Geometry: final body of the model. Coordinates: model frame, mm. Face numbers are marked on the shaded views. A direction names the side the tool comes from. Round coordinates to 2 decimals unless told otherwise and drop trailing zeros. Loops run counter-clockwise (first coordinate to the right, second up) from the corner with the lowest first, then second, coordinate; pieces in that order, holes last. Notation, with made-up numbers: (-31.75, -34) -> (-20.75, -34) arc R24 cw to (-20.75, 5) -> close; hole circle Ø3 at (43.5, 31). An arc over 180 degrees is marked (long way). Answer in a Markdown table with one row per item.
```python
from build123d import *

# Parameters (mm, degrees)
F1_DEPTH = 762
F3_DEPTH = 762.001
F4_DEPTH = 533.4
F6_DEPTH = 469.901
F8_DEPTH = 762
F7_R     = 190.5
F9_DEPTH = 762.0010001


with BuildPart() as f1:
    # F0 (on Front) → F1 (new body)
    with BuildSketch(Plane.XZ):
        with BuildLine():
            ThreePointArc((0, 6.35), (1.8598719395, 1.8598719395), (6.35, 0))
            Line((6.35, 0), (1524, 0))
            Line((1524, 0), (1524, 762))
            Line((1524, 762), (6.35, 762))
            ThreePointArc((6.35, 762), (1.8598719395, 760.1401280605), (0, 755.65))
            Line((0, 755.65), (0, 6.35))
        make_face()
    extrude(amount=F1_DEPTH)

    # F2 (on face) → F3 (cut, through all)
    with BuildSketch(Plane.XY.offset(762)):
        Polygon((1524, -228.6), (1524, 0), (1295.4, 0), align=None)
        Polygon((1524, -762), (1524, -533.4), (1295.4, -762), align=None)
    extrude(amount=-F3_DEPTH, mode=Mode.SUBTRACT)

    # F2 (on face) → F4 (cut)
    with BuildSketch(Plane.XY.offset(762)):
        Polygon((1524, -292.1), (1524, -228.6), (1295.4, 0), (457.2, 0), (457.2, -292.1), align=None)
        Polygon((1524, -533.4), (1524, -469.9), (457.2, -469.9), (457.2, -762), (1295.4, -762), align=None)
    extrude(amount=-F4_DEPTH, mode=Mode.SUBTRACT)

    # F5 (on face) → F6 (cut, through all)
    with BuildSketch(Plane.XZ.offset(469.9)):
        Polygon((1524, 762), (457.2, 762), (1524, 228.6), align=None)
    extrude(amount=-F6_DEPTH, mode=Mode.SUBTRACT)

    # F7 (on face) → F8 (join)
    with BuildSketch(Plane.XY.offset(762)):
        with BuildLine():
            Line((6.35, -190.5), (6.35, 0))
            ThreePointArc((6.35, 0), (-374.65, -381), (6.35, -762))
            Line((6.35, -762), (6.35, -571.5))
            ThreePointArc((6.35, -571.5), (-184.15, -381), (6.35, -190.5))
        make_face()
    extrude(amount=-F8_DEPTH)

    # F7 (on face) → F9 (cut, through all)
    with BuildSketch(Plane.XY.offset(762)):
        with Locations((6.35, -381)):
            Circle(F7_R)
    extrude(amount=-F9_DEPTH, mode=Mode.SUBTRACT)


solid = f1.part
```
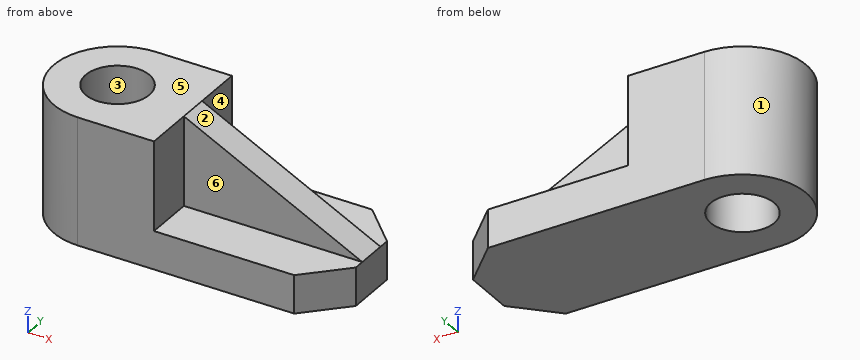
Item 1: First-contact query: P1, Ø2, axis at x = 792.5, z = 431.5, coming from the -Y side; P2, Ø3, axis at x = 1235, y = -614, coming from the +Z side; P3, Ø1, axis at y = -278, z = 478, coming from the +X side. Flat tips, straight axial feed; report the tip coordinate or a pass-through.
Ans:
| item | result |
|---|---|
| P1 | y = -469.9 |
| P2 | z = 228.6 |
| P3 | x = 457.2 |
Item 2: Section query D-D, the plane z = 546. Output: boundary loops of the cut face in (x, y).
Ans:
| item | result |
|---|---|
| outline | (0, -762) -> (457.2, -762) -> (457.2, -469.9) -> (889.2, -469.9) -> (889.2, -292.1) -> (457.2, -292.1) -> (457.2, 0) -> (0, 0) -> (0, -0.05) arc R381 ccw to (0, -761.95) -> close; hole circle Ø381 at (6.35, -381) |
Item 3: Section query B-B, the plane z = 199.5. Output: boundary loops of the cut face in (x, y).
Ans:
| item | result |
|---|---|
| outline | (0, -762) -> (1295.4, -762) -> (1524, -533.4) -> (1524, -228.6) -> (1295.4, 0) -> (0, 0) -> (0, -0.05) arc R381 ccw to (0, -761.95) -> close; hole circle Ø381 at (6.35, -381) |
Item 4: Section query C-C, the plane x = 1340.5. Output: boundary loops of the cut face in (y, z), and give its area (3 significant figures).
Ans:
| item | result |
|---|---|
| outline | (-716.9, 0) -> (-45.1, 0) -> (-45.1, 228.6) -> (-292.1, 228.6) -> (-292.1, 320.35) -> (-469.9, 320.35) -> (-469.9, 228.6) -> (-716.9, 228.6) -> close |
| area | 170,000 mm2 |
Item 5: Section query A-A, the plane y = -381. Output: boundary loops of the cut face in (x, z), and give its area (3 significant figures).
Ans:
| item | result |
|---|---|
| outline | (-374.65, 0) -> (-184.15, 0) -> (-184.15, 762) -> (-374.65, 762) -> close; (196.85, 0) -> (1524, 0) -> (1524, 228.6) -> (457.2, 762) -> (196.85, 762) -> close |
| area | 872,000 mm2 |
Item 6: Mould query, pull axis Y, two halves, no side actions, for the marked faces 1, 2 and 3. Classes: released by +Y, released by -Y, zero draft, split by the parting line, or undercut.
Ans:
| item | result |
|---|---|
| face 1 | split by the parting line |
| face 2 | zero draft |
| face 3 | undercut |
Item 7: Ray query, L1, parallel to Y at x = 6, z = 214; L2, parallel to X at y = -381, z = 214.5; L3, parallel to Z at x = 467.5, y = -609.5. Return the intervals inside material, ascending.
Ans:
| item | result |
|---|---|
| L1 | -762 to -571.5, -190.5 to 0 |
| L2 | -374.65 to -184.15, 196.85 to 1524 |
| L3 | 0 to 228.6 |
Item 8: Set-up query: the marked faces 4, 5 and 6. Return all of +Z, -Z, +X, -X, +Y, -Y with unobstructed straight access to the full face (end or side cutting, diameter ignored); none if empty.
Ans:
| item | result |
|---|---|
| face 4 | +Z, +X, +Y |
| face 5 | +Z, +X, -X, +Y, -Y |
| face 6 | +Z, +X, -Y |
